```python
from build123d import *

# Parameters (mm, degrees)
SKETCH1_R           = 2.5
BOSS_EXTRUDE1_DEPTH = 30


with BuildPart() as part:
    # Sketch1 → Boss-Extrude1 (new body)
    with BuildSketch(Plane.XY):
        with BuildLine():
            ThreePointArc((5.987788455, 46.66284585), (0, 53.045454545), (-5.987788455, 46.66284585))
            ThreePointArc((-5.987788455, 46.66284585), (-20.412257727, 42.386489922), (-32.749156909, 33.775250038))
            ThreePointArc((-32.749156909, 33.775250038), (-41.472606365, 33.073299944), (-40.215806985, 24.412366988))
            ThreePointArc((-40.215806985, 24.412366988), (-45.865926778, 10.468598484), (-46.82531916, -4.545797942))
            ThreePointArc((-46.82531916, -4.545797942), (-51.715494251, -11.803724088), (-44.160502601, -16.221122137))
            ThreePointArc((-44.160502601, -16.221122137), (-36.781617471, -29.332361133), (-25.641061021, -39.443767354))
            ThreePointArc((-25.641061021, -39.443767354), (-23.015560161, -47.792303129), (-14.851439049, -44.639775442))
            ThreePointArc((-14.851439049, -44.639775442), (0, -47.045454545), (14.851439049, -44.639775442))
            ThreePointArc((14.851439049, -44.639775442), (23.015560161, -47.792303129), (25.641061021, -39.443767354))
            ThreePointArc((25.641061021, -39.443767354), (36.781617471, -29.332361133), (44.160502601, -16.221122137))
            ThreePointArc((44.160502601, -16.221122137), (51.715494251, -11.803724088), (46.82531916, -4.545797942))
            ThreePointArc((46.82531916, -4.545797942), (45.865926778, 10.468598484), (40.215806985, 24.412366988))
            ThreePointArc((40.215806985, 24.412366988), (41.472606365, 33.073299944), (32.749156909, 33.775250038))
            ThreePointArc((32.749156909, 33.775250038), (20.412257727, 42.386489922), (5.987788455, 46.66284585))
        make_face()
        with Locations((0, 47.045454545)):
            Circle(SKETCH1_R, mode=Mode.SUBTRACT)
        with Locations((36.781617471, 29.332361133)):
            Circle(SKETCH1_R, mode=Mode.SUBTRACT)
        with Locations((45.865926778, -10.468598484)):
            Circle(SKETCH1_R, mode=Mode.SUBTRACT)
        with Locations((20.412257727, -42.386489922)):
            Circle(SKETCH1_R, mode=Mode.SUBTRACT)
        with Locations((-20.412257727, -42.386489922)):
            Circle(SKETCH1_R, mode=Mode.SUBTRACT)
        with Locations((-36.781617471, 29.332361133)):
            Circle(SKETCH1_R, mode=Mode.SUBTRACT)
        with BuildLine():
            ThreePointArc((0.677628824, -28.364607267), (21.907582959, -33.164561623), (30.469177048, -13.153324254))
            ThreePointArc((30.469177048, -13.153324254), (23.889713582, -9.599573413), (20.33596274, -16.179036879))
            ThreePointArc((20.33596274, -16.179036879), (17.098534821, -23.745961668), (9.070772057, -21.930936793))
            ThreePointArc((9.070772057, -21.930936793), (1.657365204, -20.951200413), (0.677628824, -28.364607267))
        make_face(mode=Mode.SUBTRACT)
        with BuildLine():
            ThreePointArc((24.225656049, 14.769147409), (17.767561392, 35.554804189), (-3.843475576, 32.963743483))
            ThreePointArc((-3.843475576, 32.963743483), (-3.63138235, 25.488885557), (3.843475576, 25.700978783))
            ThreePointArc((3.843475576, 25.700978783), (12.015338631, 26.680746357), (14.457362363, 18.82098743))
            ThreePointArc((14.457362363, 18.82098743), (17.315589196, 11.910920576), (24.225656049, 14.769147409))
        make_face(mode=Mode.SUBTRACT)
        with BuildLine():
            ThreePointArc((-24.903284873, 13.595459858), (-39.67514435, -2.390242566), (-26.625701472, -19.810419229))
            ThreePointArc((-26.625701472, -19.810419229), (-20.258331232, -15.889312144), (-24.179438316, -9.521941904))
            ThreePointArc((-24.179438316, -9.521941904), (-29.113873453, -2.934784689), (-23.52813442, 3.109949364))
            ThreePointArc((-23.52813442, 3.109949364), (-18.9729544, 9.040279837), (-24.903284873, 13.595459858))
        make_face(mode=Mode.SUBTRACT)
    extrude(amount=BOSS_EXTRUDE1_DEPTH)


solid = part.part
```
Source: CAD feature listing. Evaluate the final solid. Frame: model axes, mm. A direction names the side the tool comes from. Give positions to 0.01 mm unless a question says otherwise; leave off trailing zeros. Loops run counter-clockwise (first coordinate to the right, second up) from the corner with the lowest first, then second, coordinate; pieces in that order, holes last. Notation, with made-up numbers: (1, 49) -> (46, 49) arc R18 cw to (46, 73) -> close; hole circle Ø5 at (70.5, 43). An arc over 180 degrees is marked (long way). Use a Markdown table: item, result. Add a question column.
(1) First-contact query: pin 1 Ø8 at (y, z) = (-5.5, 24) entering from +X; pin 2 Ø3 at (x, y) = (-36.78, 29.33) entering from -Z; pin 3 Ø6 at (y, z) = (-23, 9.5) entering from +X; pin 4 Ø1.5 at (x, z) = (-12.5, 25.5) entering from +Y. Flat tips, straight axial feed; report the tip coordinate or a pass-through.
(2) Section query A-A (y = 7.5). Output: boundary loops of the cut face in (x, z).
(3) Ray query, line 1 (X direction, y = -42.5, z = 18.25); line 2 (X direction, y = 47, z = 7.5); line 3 (Y direction, x = 17, z = 28.75). Return the intervals inside material, ascending.
(4) Pull-direction query (X, two-part tool) for faces 1 (the face through (22.89, -47.85, 14.79)), 2 (the face through (45.913, 10.262, 14.79)), 3 (the face through (-29.12, -3.06, 14.79)); classes: +X half, -X half, draft (parallel to the pull), parting line (faces both ways), or undercut.
(5) Section query B-B (z = 26). Count the separate pieces of the cut face and the enclosed holes in it, then the cut area to 3 significant figures.
(6) Section query C-C (y = -31). Output: boundary loops of the cut face in (x, z), then the cut area to 3 significant figures.
(7) Access query for faces 4 (the face through (-0.212, -47.045, 14.79)), 5 (the face through (-39.655, -2.06, 14.79)). Directions: +Z, -Z, +X, -X, +Y, -Y. A direction counts if a zero-diameter tool reaches every point of the face in a straight line with its end or side. Return the directions, or none.
Checked values:
| question | item | result |
|---|---|---|
| 1 | pin 1 | x = 51.79 |
| 1 | pin 2 | through |
| 1 | pin 3 | x = 42.58 |
| 1 | pin 4 | y = 45.55 |
| 2 | outline | (-46.44, 0) -> (-35.86, 0) -> (-35.86, 30) -> (-46.44, 30) -> close; (-19, 0) -> (46.44, 0) -> (46.44, 30) -> (-19, 30) -> close |
| 3 | line 1 | -26.41 to -22.91, -17.91 to 17.91, 22.91 to 26.41 |
| 3 | line 2 | -6 to -2.5, 2.5 to 6 |
| 3 | line 3 | -47.32 to -34.79, -23.8 to 12.05, 36.02 to 43.87 |
| 4 | face 1 | undercut |
| 4 | face 2 | +X half |
| 4 | face 3 | undercut |
| 5 | separate pieces | 1 |
| 5 | enclosed holes | 9 |
| 5 | area | 5,950 mm^2 |
| 6 | outline | (-35.39, 0) -> (3.19, 0) -> (3.19, 30) -> (-35.39, 30) -> close; (25.16, 0) -> (35.39, 0) -> (35.39, 30) -> (25.16, 30) -> close |
| 6 | area | 1,460 mm^2 |
| 7 | face 4 | +Z, -Z, -Y |
| 7 | face 5 | +Z, -Z |
